```python
from build123d import *

# Parameters (mm, degrees)
F0_W     = 63.5
F0_H     = 50.8
F4_DEPTH = 76.201


# Not quite as in the source:
# - a fillet or chamfer that OpenCascade refuses, or shapes differently, is made with other operations: its cross-section is extruded or revolved along the edge and cut away or added


with BuildPart() as f1:
    # F0 (on Front) → F1 (revolve)
    with BuildSketch(Plane.XZ):
        with Locations((57.15, 25.4)):
            Rectangle(F0_W, F0_H)
    revolve(axis=Axis((0, 0, 63.5), (0, 0, 1)))

    # F3 (on offset) → F4 (cut, through all)
    with BuildSketch(Plane.XY.offset(76.2)):
        with BuildLine():
            ThreePointArc((0, 76.2), (3.175, 76.1338254326), (6.3444854527, 75.9354166667))
            ThreePointArc((6.3444854527, 75.9354166667), (6.3486212135, 76.0676796024), (6.35, 76.2))
            ThreePointArc((6.35, 76.2), (-0.1323203976, 82.5486212135), (-6.3444854527, 75.9354166667))
            ThreePointArc((-6.3444854527, 75.9354166667), (-3.175, 76.1338254326), (0, 76.2))
        make_face()
        with BuildLine():
            Line((0, 69.85), (0, 76.2))
            ThreePointArc((0, 76.2), (-3.175, 76.1338254326), (-6.3444854527, 75.9354166667))
            ThreePointArc((-6.3444854527, 75.9354166667), (-4.3955884608, 71.6172822383), (0, 69.85))
        make_face()
        with BuildLine():
            ThreePointArc((0, 69.85), (4.3955884608, 71.6172822383), (6.3444854527, 75.9354166667))
            ThreePointArc((6.3444854527, 75.9354166667), (3.175, 76.1338254326), (0, 76.2))
            Line((0, 76.2), (0, 69.85))
        make_face()
        with BuildLine():
            ThreePointArc((62.5897571539, 43.4621939093), (65.9911357684, 38.1), (68.9342426066, 32.4732227573))
            ThreePointArc((68.9342426066, 32.4732227573), (71.4230428194, 34.8110965675), (72.3411357684, 38.1))
            ThreePointArc((72.3411357684, 38.1), (69.0508535493, 43.6642274487), (62.5897571539, 43.4621939093))
        make_face()
        with BuildLine():
            ThreePointArc((62.5897571539, 43.4621939093), (60.4918744543, 34.925), (68.9342426066, 32.4732227573))
            ThreePointArc((68.9342426066, 32.4732227573), (65.9911357684, 38.1), (62.5897571539, 43.4621939093))
        make_face()
        with BuildLine():
            ThreePointArc((62.5897571539, -43.4621939093), (65.9911357684, -38.1), (68.9342426066, -32.4732227573))
            ThreePointArc((68.9342426066, -32.4732227573), (60.4918744543, -34.925), (62.5897571539, -43.4621939093))
        make_face()
        with BuildLine():
            ThreePointArc((72.3411357684, -38.1), (71.4230428194, -34.8110965675), (68.9342426066, -32.4732227573))
            ThreePointArc((68.9342426066, -32.4732227573), (65.9911357684, -38.1), (62.5897571539, -43.4621939093))
            ThreePointArc((62.5897571539, -43.4621939093), (69.0508535493, -43.6642274487), (72.3411357684, -38.1))
        make_face()
        with BuildLine():
            ThreePointArc((-6.3444854527, -75.9354166667), (0, -76.2), (6.3444854527, -75.9354166667))
            ThreePointArc((6.3444854527, -75.9354166667), (0, -69.85), (-6.3444854527, -75.9354166667))
        make_face()
        with BuildLine():
            ThreePointArc((6.35, -76.2), (6.3486212135, -76.0676796024), (6.3444854527, -75.9354166667))
            ThreePointArc((6.3444854527, -75.9354166667), (0, -76.2), (-6.3444854527, -75.9354166667))
            ThreePointArc((-6.3444854527, -75.9354166667), (-0.1323203976, -82.5486212135), (6.35, -76.2))
        make_face()
        with BuildLine():
            ThreePointArc((-68.9342426066, -32.4732227573), (-71.4903970824, -41.275), (-62.5897571539, -43.4621939093))
            ThreePointArc((-62.5897571539, -43.4621939093), (-65.9911357684, -38.1), (-68.9342426066, -32.4732227573))
        make_face()
        with BuildLine():
            ThreePointArc((-68.9342426066, -32.4732227573), (-65.9911357684, -38.1), (-62.5897571539, -43.4621939093))
            ThreePointArc((-62.5897571539, -43.4621939093), (-60.4269083197, -41.159717781), (-59.6411357684, -38.1))
            ThreePointArc((-59.6411357684, -38.1), (-62.7022323358, -32.6680929489), (-68.9342426066, -32.4732227573))
        make_face()
        with BuildLine():
            ThreePointArc((-68.9342426066, 32.4732227573), (-65.9911357684, 38.1), (-62.5897571539, 43.4621939093))
            ThreePointArc((-62.5897571539, 43.4621939093), (-71.4903970824, 41.275), (-68.9342426066, 32.4732227573))
        make_face()
        with BuildLine():
            ThreePointArc((-59.6411357684, 38.1), (-60.4269083197, 41.159717781), (-62.5897571539, 43.4621939093))
            ThreePointArc((-62.5897571539, 43.4621939093), (-65.9911357684, 38.1), (-68.9342426066, 32.4732227573))
            ThreePointArc((-68.9342426066, 32.4732227573), (-62.7022323358, 32.6680929489), (-59.6411357684, 38.1))
        make_face()
    extrude(amount=-F4_DEPTH, mode=Mode.SUBTRACT)

    # F5: fillet of radius 12.7 on 1 edges, made by hand

    # F5_s1 → F5_t2 (revolve, cut)
    with BuildSketch(Plane.XZ):
        with BuildLine():
            ThreePointArc((76.2, 50.8), (85.1802561211, 47.0802561211), (88.9, 38.1))
            Line((88.9, 38.1), (88.9, 50.8))
            Line((88.9, 50.8), (76.2, 50.8))
        make_face()
    revolve(axis=Axis((0, 0, 50.8), (0, 0, 1)), mode=Mode.SUBTRACT)

    # F6: chamfer of 12.7 on 3 edges, made by hand

    # F6_s1 → F6_t2 (revolve, cut)
    with BuildSketch(Plane.XZ):
        Polygon((76.2, 0), (88.9, 12.7), (88.9, 0), align=None)
    revolve(axis=Axis((0, 0, 0), (0, 0, 1)), mode=Mode.SUBTRACT)


solid = f1.part
```
Work out the finished part from the listing and answer in its coordinate system (mm). Coordinates: 2 decimals unless noted, no trailing zeros. Order: outer loops, then holes, each group sorted by start corner. A loop starts at its lowest first (then second) coordinate and runs counter-clockwise, first axis right, second up. Notation, with made-up numbers: (42, -1.75) - (47, -1.75) arc R13 cw to (47, 20.25) - close; hole circle Ø9 at (6.5, 9). An arc over 180 degrees is marked (long way). Answer as a JSON object with one key per item and string values.
1. Find section C-C on x = -65. Count the separate pieces of the cut face and the enclosed holes in it, plus the area to 3 significant figures.
Output values:
{"separate pieces": "3", "enclosed holes": "0", "area": "4,540 mm²"}
2. Each of these flat-tipped pins is pushed along its axis until it touches: P1, Ø6, axis at y = -16.5, z = 45.5, coming from the -X side; P2, Ø4, axis at x = -51, y = 57.5, coming from the +Z side; P3, Ø5, axis at y = -36.5, z = 17.5, coming from the +X side; P4, Ø12, axis at y = -17.5, z = 25.5, coming from the -X side. Where does it stop, or does it pass through?
Output values:
{"P1": "stops at x = -86.68", "P2": "stops at z = 50.8", "P3": "stops at x = 82.14", "P4": "stops at x = -88.15"}
3. Find section B-B on z = 34. Determine the outline of the cut face in (x, y), plus the area to 3 significant figures.
Output values:
{"outline": "circle Ø177.8 at (0, 0); hole circle Ø12.7 at (-65.99, -38.1); hole circle Ø12.7 at (-65.99, 38.1); hole circle Ø50.8 at (0, 0); hole circle Ø12.7 at (0, -76.2); hole circle Ø12.7 at (0, 76.2); hole circle Ø12.7 at (65.99, -38.1); hole circle Ø12.7 at (65.99, 38.1)", "area": "22,000 mm²"}
4. Find section A-A on y = 0. Determine the outline of the cut face in (x, z).
Output values:
{"outline": "(-88.9, 12.7) - (-76.2, 0) - (-25.4, 0) - (-25.4, 50.8) - (-76.2, 50.8) arc R12.7 ccw to (-88.9, 38.1) - close; (25.4, 0) - (76.2, 0) - (88.9, 12.7) - (88.9, 38.1) arc R12.7 ccw to (76.2, 50.8) - (25.4, 50.8) - close"}
5. Consider line 1 (X direction, y = -38.1, z = 28.5); line 2 (Y direction, x = 0.5, z = 23); line 3 (Y direction, x = 61, z = 38). Determine where each line is inside the solid, lowest interval first.
Output values:
{"line 1": "x = -80.32 to -72.34, -59.64 to 59.64, 72.34 to 80.32", "line 2": "y = -88.9 to -82.53, -69.87 to -25.4, 25.4 to 69.87, 82.53 to 88.9", "line 3": "y = -64.67 to -42.03, -34.17 to 34.17, 42.03 to 64.67"}
